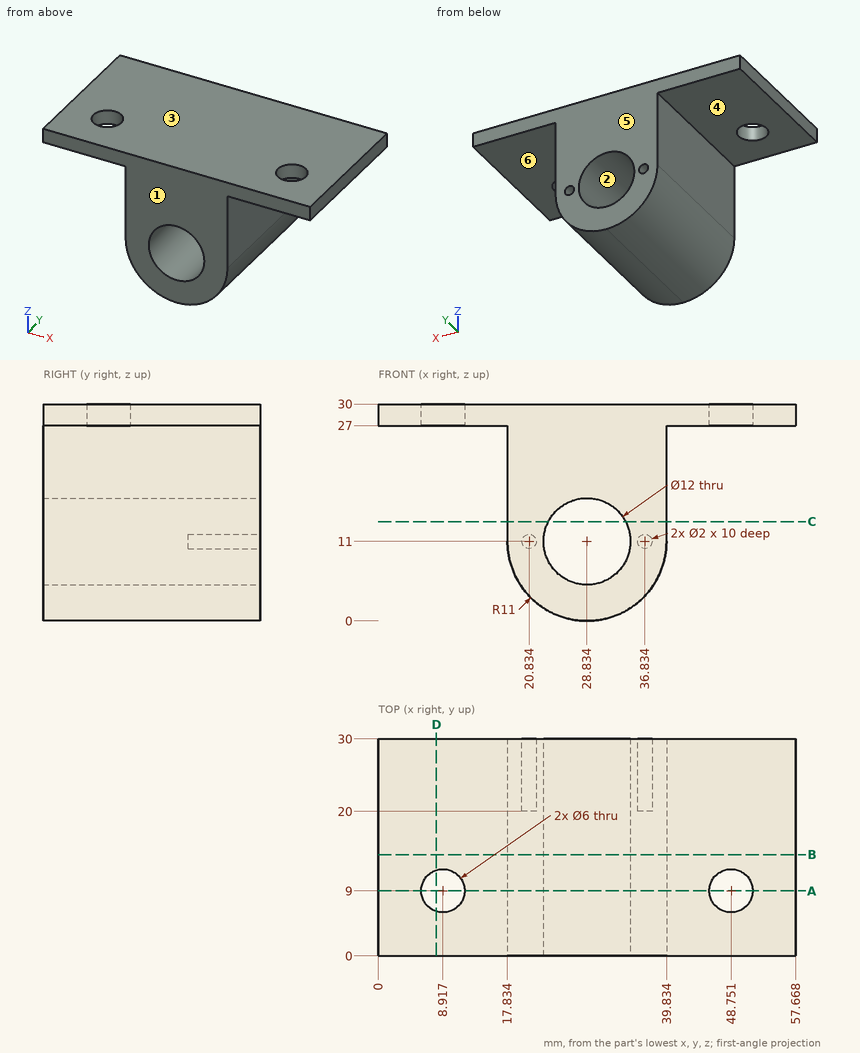
For this review, use the dimensioned drawing (mm, ordinates from the lowest corner) and the shaded views. A direction names the side the tool comes from. Coordinates: 2 decimals unless noted, no trailing zeros. Loops run counter-clockwise (first coordinate to the right, second up) from the corner with the lowest first, then second, coordinate; pieces in that order, holes last. Notation, with made-up numbers: (30.5, -32.75) -> (56.5, -32.75) arc R22 ccw to (56.5, -14.75) -> close; hole circle Ø9 at (82, 49). An arc over 180 degrees is marked (long way). Use a Markdown table: item, result. Add a question column.
Item 1: We need section B-B, the plane y = 14. Write out the cut boundary in (x, z), and give its area (3 significant figures).
Item 2: We need section A-A, the plane y = 9. Write out the cut boundary in (x, z).
Item 3: Clearance check with flat-ended pins moving along their axes: P1, Ø14.5, axis at x = 49, y = 22.5, coming from the -Z side; P2, Ø0.6, axis at x = 36.5, z = 11, coming from the +Y side; P3, Ø5, axis at x = 8.92, y = 9, coming from the +Z side; P4, Ø13, axis at y = 12, z = 19, coming from the +X side. State where each tip first meets the part, or that it passes through.
Item 4: The part is to be moulded in two halves that separate along Z. For the marked faces 1, 2 and 3, say which applies: +Z half, -Z half, draft (parallel to the pull), parting line (faces both ways), or undercut.
Item 5: We need section C-C, the plane z = 13.75. Write out the cut boundary in (x, y).
Item 6: Machinability: for the marked faces 4, 5 and 6, which of the approach directions +Z, -Z, +X, -X, +Y, -Y give a long, thin tool a straight path to every point of the face, cutting with its end or side? Answer none if there is none.
Item 7: Wall thickness on L1, parallel to Z at x = 17, y = 17.5; L2, parallel to X at y = 23.25, z = 23.25; L3, parallel to X at y = 16, z = 8.5: over which ranges is each line inside the solid? List them lowest first. Write a range as from..to.
Item 8: We need section D-D, the plane x = 8. Write out the cut boundary in (y, z).
Numbers:
| question | item | result |
|---|---|---|
| 1 | outline | (0, 27) -> (17.83, 27) -> (17.83, 11) arc R11 ccw to (39.83, 11) -> (39.83, 27) -> (57.67, 27) -> (57.67, 30) -> (0, 30) -> close; hole circle Ø12 at (28.83, 11) |
| 1 | area | 602 mm^2 |
| 2 | outline | (0, 27) -> (5.92, 27) -> (5.92, 30) -> (0, 30) -> close; (11.92, 27) -> (17.83, 27) -> (17.83, 11) arc R11 ccw to (39.83, 11) -> (39.83, 27) -> (45.75, 27) -> (45.75, 30) -> (11.92, 30) -> close; (51.75, 27) -> (57.67, 27) -> (57.67, 30) -> (51.75, 30) -> close; hole circle Ø12 at (28.83, 11) |
| 3 | P1 | stops at z = 27 |
| 3 | P2 | stops at y = 20 |
| 3 | P3 | passes through |
| 3 | P4 | stops at x = 39.83 |
| 4 | face 1 | draft |
| 4 | face 2 | undercut |
| 4 | face 3 | +Z half |
| 5 | outline | (17.83, 0) -> (23.5, 0) -> (23.5, 30) -> (17.83, 30) -> close; (34.17, 0) -> (39.83, 0) -> (39.83, 30) -> (34.17, 30) -> close |
| 6 | face 4 | -Z, -X, +Y, -Y |
| 6 | face 5 | +Z, -Z, +X, -X, +Y |
| 6 | face 6 | -Z, +X, +Y, -Y |
| 7 | L1 | z = 27..30 |
| 7 | L2 | x = 17.83..39.83 |
| 7 | L3 | x = 18.12..23.38, 34.29..39.55 |
| 8 | outline | (0, 27) -> (6.14, 27) -> (6.14, 30) -> (0, 30) -> close; (11.86, 27) -> (30, 27) -> (30, 30) -> (11.86, 30) -> close |
